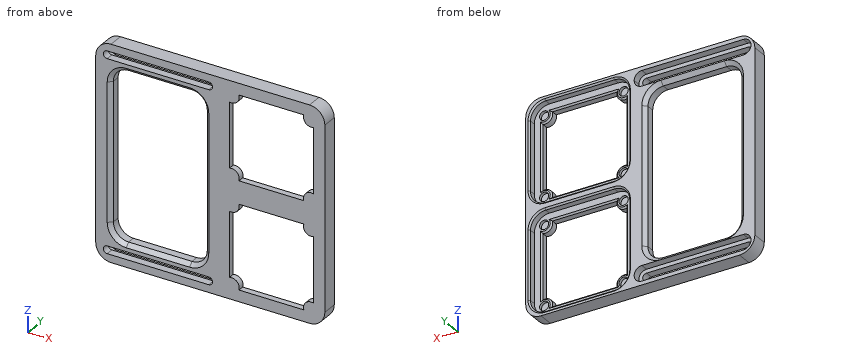
```python
from build123d import *

# Parameters (mm, degrees)
SKETCH1_W           = 70
SKETCH1_H           = 70
BOSS_EXTRUDE2_DEPTH = 7
CUT_EXTRUDE1_DEPTH  = 5
SKETCH9_W           = 70
SKETCH9_H           = 70
BOSS_EXTRUDE3_DEPTH = 5
CUT_EXTRUDE11_DEPTH = 100.242128151
SKETCH21_R          = 3
CUT_EXTRUDE12_DEPTH = 2
CHAMFER3_SIZE       = 1
CUT_EXTRUDE13_START = -2
SKETCH22_W          = 70
SKETCH22_H          = 70
CUT_EXTRUDE13_DEPTH = 2
FILLET1_R           = 10
SKETCH23_W          = 140
SKETCH23_H          = 10
BOSS_EXTRUDE4_DEPTH = 80
CUT_EXTRUDE14_DEPTH = 70
FILLET2_R           = 10
CUT_EXTRUDE15_DEPTH = 70
CHAMFER5_SIZE       = 2.5
CUT_EXTRUDE16_DEPTH = 5
CUT_EXTRUDE17_DEPTH = 5


with BuildPart() as part:
    # Sketch1 → Boss-Extrude2 (new body)
    with BuildSketch(Plane(origin=(0, 0, 0), x_dir=(1, 0, 0), z_dir=(0, 1, 0))):
        with Locations((35, 35)):
            Rectangle(SKETCH1_W, SKETCH1_H)
    extrude(amount=BOSS_EXTRUDE2_DEPTH)

    # Sketch3 → Cut-Extrude1 (cut)
    with BuildSketch(Plane(origin=(0, 7, 0), x_dir=(1, 0, 0), z_dir=(0, 1, 0))):
        with BuildLine():
            Line((2.5, 57.5), (2.5, 12.5))
            ThreePointArc((2.5, 12.5), (5.428932188, 5.428932188), (12.5, 2.5))
            Line((12.5, 2.5), (57.5, 2.5))
            ThreePointArc((57.5, 2.5), (64.571067812, 5.428932188), (67.5, 12.5))
            Line((67.5, 12.5), (67.5, 57.5))
            ThreePointArc((67.5, 57.5), (64.571067812, 64.571067812), (57.5, 67.5))
            Line((57.5, 67.5), (12.5, 67.5))
            ThreePointArc((12.5, 67.5), (5.428932188, 64.571067812), (2.5, 57.5))
        make_face()
    extrude(amount=-CUT_EXTRUDE1_DEPTH, mode=Mode.SUBTRACT)

    # Sketch9 → Boss-Extrude3 (add)
    with BuildSketch(Plane.XZ):
        with Locations((35, -35)):
            Rectangle(SKETCH9_W, SKETCH9_H)
    extrude(amount=BOSS_EXTRUDE3_DEPTH)

    # Sketch20 → Cut-Extrude11 (cut, through all)
    with BuildSketch(Plane(origin=(0, 2, 0), x_dir=(1, 0, 0), z_dir=(0, 1, 0))):
        with BuildLine():
            Line((13.745191882, 7.5), (56.254808118, 7.5))
            ThreePointArc((56.254808118, 7.5), (57.5, 12.5), (62.5, 13.745191882))
            Line((62.5, 13.745191882), (62.5, 56.254808118))
            ThreePointArc((62.5, 56.254808118), (57.5, 57.5), (56.254808118, 62.5))
            Line((56.254808118, 62.5), (13.745191882, 62.5))
            ThreePointArc((13.745191882, 62.5), (12.5, 57.5), (7.5, 56.254808118))
            Line((7.5, 56.254808118), (7.5, 13.745191882))
            ThreePointArc((7.5, 13.745191882), (12.5, 12.5), (13.745191882, 7.5))
        make_face()
    extrude(amount=-CUT_EXTRUDE11_DEPTH, mode=Mode.SUBTRACT)

    # Sketch21 → Cut-Extrude12 (cut)
    with BuildSketch(Plane(origin=(0, 2, 0), x_dir=(1, 0, 0), z_dir=(0, 1, 0))):
        with Locations(Location((8.964466094, 61.035533906, 0), (0, 0, 270))):
            Circle(SKETCH21_R)
        with Locations(Location((61.035533906, 61.035533906, 0), (0, 0, 270))):
            Circle(SKETCH21_R)
        with Locations(Location((61.035533906, 8.964466094, 0), (0, 0, 270))):
            Circle(SKETCH21_R)
        with Locations(Location((8.964466094, 8.964466094, 0), (0, 0, 270))):
            Circle(SKETCH21_R)
    extrude(amount=-CUT_EXTRUDE12_DEPTH, mode=Mode.SUBTRACT)

    # Chamfer3
    chamfer3_edges = [part.edges().sort_by_distance(p)[0] for p in [
        (5.428932188, 7, -5.428932188),
        (35, 7, -2.5),
        (64.571067812, 7, -5.428932188),
        (67.5, 7, -35),
        (64.571067812, 7, -64.571067812),
        (35, 7, -67.5),
        (5.428932188, 7, -64.571067812),
        (2.5, 7, -35),
        (12.5, 2, -12.5),
        (12.5, 2, -57.5),
        (57.5, 2, -57.5),
        (57.5, 2, -12.5),
        (35, 2, -7.5),
        (62.5, 2, -35),
        (35, 2, -62.5),
        (7.5, 2, -35),
    ]]
    chamfer(chamfer3_edges, length=CHAMFER3_SIZE)

    # Sketch22 → Cut-Extrude13 (cut)
    with BuildSketch(Plane.XZ.offset(5).offset(CUT_EXTRUDE13_START)):
        with Locations((35, -35)):
            Rectangle(SKETCH22_W, SKETCH22_H)
        with BuildLine():
            Line((7.5, -13.745191882), (7.5, -56.254808118))
            ThreePointArc((7.5, -56.254808118), (12.5, -57.5), (13.745191882, -62.5))
            Line((13.745191882, -62.5), (56.254808118, -62.5))
            ThreePointArc((56.254808118, -62.5), (57.5, -57.5), (62.5, -56.254808118))
            Line((62.5, -56.254808118), (62.5, -13.745191882))
            ThreePointArc((62.5, -13.745191882), (57.5, -12.5), (56.254808118, -7.5))
            Line((56.254808118, -7.5), (13.745191882, -7.5))
            ThreePointArc((13.745191882, -7.5), (12.5, -12.5), (7.5, -13.745191882))
        make_face(mode=Mode.SUBTRACT)
    extrude(amount=CUT_EXTRUDE13_DEPTH, mode=Mode.SUBTRACT)

    # Mirror2: part across plane


with BuildPart() as part_1:
    add(part.part)
    add(part.part.mirror(Plane(origin=(0, 7, -70), x_dir=(1, 0, 0), z_dir=(0, 0, 1))))

    # Fillet1
    fillet1_edges = [part_1.edges().sort_by_distance(p)[0] for p in [
        (70, 2, -140),
        (70, 2, 0),
    ]]
    fillet(fillet1_edges, radius=FILLET1_R)

    # Sketch23 → Boss-Extrude4 (add)
    with BuildSketch(Plane.ZY):
        with Locations((-70, 2)):
            Rectangle(SKETCH23_W, SKETCH23_H)
    extrude(amount=BOSS_EXTRUDE4_DEPTH)

    # Sketch24 → Cut-Extrude14 (cut)
    with BuildSketch(Plane(origin=(0, 7, 0), x_dir=(1, 0, 0), z_dir=(0, 1, 0))):
        with BuildLine():
            Line((-72.5, 5), (-6, 5))
            ThreePointArc((-6, 5), (-3.5, 7.5), (-6, 10))
            Line((-6, 10), (-72.5, 10))
            ThreePointArc((-72.5, 10), (-75, 7.5), (-72.5, 5))
        make_face()
        with BuildLine():
            Line((-72.5, 135), (-6, 135))
            ThreePointArc((-6, 135), (-3.5, 132.5), (-6, 130))
            Line((-6, 130), (-72.5, 130))
            ThreePointArc((-72.5, 130), (-75, 132.5), (-72.5, 135))
        make_face()
    extrude(amount=-CUT_EXTRUDE14_DEPTH, mode=Mode.SUBTRACT)

    # Fillet2
    fillet2_edges = [part_1.edges().sort_by_distance(p)[0] for p in [
        (-80, 2, -140),
        (-80, 2, 0),
    ]]
    fillet(fillet2_edges, radius=FILLET2_R)

    # Sketch25 → Cut-Extrude15 (cut)
    with BuildSketch(Plane(origin=(0, 7, 0), x_dir=(1, 0, 0), z_dir=(0, 1, 0))):
        with BuildLine():
            Line((-70, 25), (-70, 115))
            ThreePointArc((-70, 115), (-67.071067812, 122.071067812), (-60, 125))
            Line((-60, 125), (-18.5, 125))
            ThreePointArc((-18.5, 125), (-11.428932188, 122.071067812), (-8.5, 115))
            Line((-8.5, 115), (-8.5, 25))
            ThreePointArc((-8.5, 25), (-11.428932188, 17.928932188), (-18.5, 15))
            Line((-18.5, 15), (-60, 15))
            ThreePointArc((-60, 15), (-67.071067812, 17.928932188), (-70, 25))
        make_face()
    extrude(amount=-CUT_EXTRUDE15_DEPTH, mode=Mode.SUBTRACT)

    # Chamfer5
    chamfer5_edges = [part_1.edges().sort_by_distance(p)[0] for p in [
        (-3.5, 7, -7.5),
        (-75, 7, -7.5),
        (-39.25, 7, -10),
        (-39.25, 7, -5),
        (-39.25, 7, -135),
        (-39.25, 7, -130),
        (-3.5, 7, -132.5),
        (-75, 7, -132.5),
        (-67.071067812, -3, -17.928932188),
        (-39.25, -3, -15),
        (-11.428932188, -3, -17.928932188),
        (-8.5, -3, -70),
        (-11.428932188, -3, -122.071067812),
        (-39.25, -3, -125),
        (-67.071067812, -3, -122.071067812),
        (-70, -3, -70),
        (-70, 7, -70),
        (-67.071067812, 7, -122.071067812),
        (-39.25, 7, -125),
        (-11.428932188, 7, -122.071067812),
        (-8.5, 7, -70),
        (-11.428932188, 7, -17.928932188),
        (-39.25, 7, -15),
        (-67.071067812, 7, -17.928932188),
    ]]
    chamfer(chamfer5_edges, length=CHAMFER5_SIZE - 0.0001)  # a hair under: the kernel refuses the full size

    # Sketch26 → Cut-Extrude16 (cut)
    with BuildSketch(Plane(origin=(0, 7, 0), x_dir=(1, 0, 0), z_dir=(0, 1, 0))):
        with BuildLine():
            ThreePointArc((-72.5, 137.5), (-77.5, 132.5), (-72.5, 127.5))
            ThreePointArc((-72.5, 127.5), (-68.964466094, 128.964466094), (-67.5, 132.5))
            ThreePointArc((-67.5, 132.5), (-68.964466094, 136.035533906), (-72.5, 137.5))
        make_face()
        with BuildLine():
            ThreePointArc((-67.5, 132.5), (-68.964466094, 128.964466094), (-72.5, 127.5))
            Line((-72.5, 127.5), (-60, 127.5))
            Line((-60, 127.5), (-18.5, 127.5))
            Line((-18.5, 127.5), (-6, 127.5))
            ThreePointArc((-6, 127.5), (-11, 132.5), (-6, 137.5))
            Line((-6, 137.5), (-72.5, 137.5))
            ThreePointArc((-72.5, 137.5), (-68.964466094, 136.035533906), (-67.5, 132.5))
        make_face()
        with BuildLine():
            Line((-6, 127.5), (-6, 137.5))
            ThreePointArc((-6, 137.5), (-1, 132.5), (-6, 127.5))
        make_face()
        with BuildLine():
            ThreePointArc((-1, 132.5), (-2.464466094, 136.035533906), (-6, 137.5))
            Line((-6, 137.5), (-6, 127.5))
            ThreePointArc((-6, 127.5), (-2.464466094, 128.964466094), (-1, 132.5))
        make_face()
        with BuildLine():
            Line((-6, 127.5), (-6, 137.5))
            ThreePointArc((-6, 137.5), (-11, 132.5), (-6, 127.5))
        make_face()
    extrude(amount=-CUT_EXTRUDE16_DEPTH, mode=Mode.SUBTRACT)

    # Sketch27 → Cut-Extrude17 (cut)
    with BuildSketch(Plane(origin=(0, 7, 0), x_dir=(1, 0, 0), z_dir=(0, 1, 0))):
        with BuildLine():
            ThreePointArc((-6, 12.5), (-11, 7.5), (-6, 2.5))
            Line((-6, 2.5), (-6, 12.5))
        make_face()
        with BuildLine():
            Line((-6, 12.5), (-6, 2.5))
            ThreePointArc((-6, 2.5), (-2.464466094, 3.964466094), (-1, 7.5))
            ThreePointArc((-1, 7.5), (-2.464466094, 11.035533906), (-6, 12.5))
        make_face()
        with BuildLine():
            Line((-6, 12.5), (-6, 2.5))
            ThreePointArc((-6, 2.5), (-1, 7.5), (-6, 12.5))
        make_face()
        with BuildLine():
            Line((-60, 12.5), (-72.5, 12.5))
            ThreePointArc((-72.5, 12.5), (-68.964466094, 11.035533906), (-67.5, 7.5))
            ThreePointArc((-67.5, 7.5), (-68.964466094, 3.964466094), (-72.5, 2.5))
            Line((-72.5, 2.5), (-6, 2.5))
            ThreePointArc((-6, 2.5), (-11, 7.5), (-6, 12.5))
            Line((-6, 12.5), (-18.5, 12.5))
            Line((-18.5, 12.5), (-60, 12.5))
        make_face()
        with BuildLine():
            ThreePointArc((-67.5, 7.5), (-68.964466094, 11.035533906), (-72.5, 12.5))
            ThreePointArc((-72.5, 12.5), (-77.5, 7.5), (-72.5, 2.5))
            ThreePointArc((-72.5, 2.5), (-68.964466094, 3.964466094), (-67.5, 7.5))
        make_face()
    extrude(amount=-CUT_EXTRUDE17_DEPTH, mode=Mode.SUBTRACT)


solid = part_1.part
```
The listing builds one solid part. Answer for the finished solid, in the listing's coordinates (mm). Round coordinates to 2 decimals unless told otherwise and drop trailing zeros. Loops run counter-clockwise (first coordinate to the right, second up) from the corner with the lowest first, then second, coordinate; pieces in that order, holes last.
Q1. Find the intervals of material crossed by line 1 (Z direction, x = -54, y = 3); line 2 (Z direction, x = 57, y = 3.5); line 3 (Z direction, x = 44, y = 0), in increasing order.
Q2. Section A-A, the plane z = -105 is taken. Determine the outline of the cut face in (x, y), then the cut area to 3 significant figures.
Q3. Section B-B, the plane x = 25 is taken. Determine the outline of the cut face in (y, z).
Q4. Section C-C, the plane x = -12 is taken. Count the separate pieces of the cut face and the enclosed holes in it, then the cut area to 3 significant figures.
Q5. Given pin 1 Ø1.8 at (x, z) = (61, -9.5) entering from +Y; pin 2 Ø6.5 at (x, z) = (61.5, -129.5) entering from +Y, each flat-ended and moving along its own axis, determine where each tip first touches the part or whether it passes through.
Completed:
1. line 1: z = -140 to -137.5, -127.5 to -125, -15 to -12.5, -2.5 to 0
1. line 2: z = -140 to -137.5, -72.5 to -67.5, -2.5 to 0
1. line 3: z = -140 to -132.5, -77.5 to -62.5, -7.5 to 0
2. outline: (-80, -3) - (-72.5, -3) - (-70, -0.5) - (-70, 4.5) - (-72.5, 7) - (-80, 7) - close; (-8.5, -0.5) - (-6, -3) - (7.5, -3) - (7.5, 1) - (6.5, 2) - (2.5, 2) - (2.5, 6) - (1.5, 7) - (-6, 7) - (-8.5, 4.5) - close; (62.5, -3) - (70, -3) - (70, 7) - (68.5, 7) - (67.5, 6) - (67.5, 2) - (63.5, 2) - (62.5, 1) - close
2. area: 271 mm2
3. outline: (-3, -140) - (7, -140) - (7, -138.5) - (6, -137.5) - (2, -137.5) - (2, -133.5) - (1, -132.5) - (-3, -132.5) - close; (-3, -77.5) - (1, -77.5) - (2, -76.5) - (2, -72.5) - (6, -72.5) - (7, -71.5) - (7, -68.5) - (6, -67.5) - (2, -67.5) - (2, -63.5) - (1, -62.5) - (-3, -62.5) - close; (-3, -7.5) - (1, -7.5) - (2, -6.5) - (2, -2.5) - (6, -2.5) - (7, -1.5) - (7, 0) - (-3, 0) - close
4. separate pieces: 4
4. enclosed holes: 0
4. area: 182 mm2
5. pin 1: stops at y = 0
5. pin 2: stops at y = 2
